Design review of the part built by this model. Coordinates are the model's own, in mm. A direction names the side the tool comes from. Give positions to 0.01 mm unless a question says otherwise; leave off trailing zeros. Write each loop counter-clockwise with the first axis right and the second up, starting at its lowest first coordinate (ties: lowest second). Pieces come first, ordered by that corner, then holes. Notation, with made-up numbers: M 3.5,89.25 L 42.5,89.25 A19 cw 42.5,117.25 Z; hole C 13,-12 d5. An arc over 180 degrees is marked long. Write each question's results on one line, items separated by ' | '. Start each with the question number.
from build123d import *

# Parameters (mm, degrees)
SKETCH2_W               = 900
SKETCH2_H               = 300
BOSS_EXTRUDE1_DEPTH     = 600
CUT_EXTRUDE1_DEPTH      = 1
CUT_EXTRUDE1_DEPTH_BACK = 900
CUT_EXTRUDE2_DEPTH      = 1
CUT_EXTRUDE2_DEPTH_BACK = 598.5
SKETCH6_W               = 897
SKETCH6_H               = 597
CUT_EXTRUDE4_DEPTH      = 48.5


with BuildPart() as part:
    # Sketch2 → Boss-Extrude1 (new body)
    with BuildSketch(Plane.XY):
        with Locations((75.531914894, 52.659574468)):
            Rectangle(SKETCH2_W, SKETCH2_H)
    extrude(amount=-BOSS_EXTRUDE1_DEPTH)

    # Sketch3 → Cut-Extrude1 (cut, two sides)
    with BuildSketch(Plane.ZY.offset(374.468085106)) as cut_extrude1_sk:
        Polygon((-1951.6407865, 202.659574468), (-600, 202.659574468), (-598.5, 202.659574468), (-598.5, 52.659574468), (0, 52.659574468), (1351.6407865, 52.659574468), (1474.268787585, 2753.15834993), (-1829.012785414, 2903.15834993), align=None)
    extrude(amount=CUT_EXTRUDE1_DEPTH, mode=Mode.SUBTRACT)
    extrude(cut_extrude1_sk.sketch, amount=-CUT_EXTRUDE1_DEPTH_BACK, mode=Mode.SUBTRACT)

    # Sketch4 → Cut-Extrude2 (cut, two sides)
    with BuildSketch(Plane.XY) as cut_extrude2_sk:
        Polygon((-2209.296844196, 52.659574468), (-374.468085106, 52.659574468), (-372.968085106, 52.659574468), (-372.968085106, -47.340425532), (524.031914894, -47.340425532), (524.031914894, 52.659574468), (525.531914894, 52.659574468), (2360.360673983, 52.659574468), (2360.360673983, 3722.317092647), (-2209.296844196, 3722.317092647), align=None)
    extrude(amount=CUT_EXTRUDE2_DEPTH, mode=Mode.SUBTRACT)
    extrude(cut_extrude2_sk.sketch, amount=-CUT_EXTRUDE2_DEPTH_BACK, mode=Mode.SUBTRACT)

    # Sketch6 → Cut-Extrude4 (cut)
    with BuildSketch(Plane(origin=(0, -47.340425532, 0), x_dir=(1, 0, 0), z_dir=(0, 1, 0))):
        with Locations((75.531914894, 300)):
            Rectangle(SKETCH6_W, SKETCH6_H)
    extrude(amount=-CUT_EXTRUDE4_DEPTH, mode=Mode.SUBTRACT)


solid = part.part
Q1. For pin 1 Ø1.2 at (x, z) = (-374, -239) entering from +Y; pin 2 Ø0.8 at (x, z) = (-17.5, -0.5) entering from +Y; pin 3 Ø1 at (x, z) = (256.5, -401.5) entering from +Y, all flat-tipped, find the tip position at first contact; note any pin that passes through.
Q2. We need section D-D on y = 139. Write out the cut boundary in (x, z).
Q3. The part is to be moulded in two halves that separate along X. For faces 1 (the flat face through (69, -95.84, -304)), 2 (the flat face through (525.532, -16, -296)), 3 (the flat face through (69, -97.34, -296)), say which applies: pulls with the +X half, pulls with the -X half, needs draft (parallel to the pull), parting line crosses it, or undercut.
Q4. Wall thickness on line 1 along X through (y, z) = (11, -353); line 2 along Z through (x, y) = (-227.5, -83); line 3 along Y through (x, z) = (48, -434.5): over which ranges is each line inside the solid? List them lowest first. Write a range as from..to.
Q5. We need section A-A on z = -544. Write out the cut boundary in (x, y), and give its area (3 significant figures).
Q6. We need section C-C on y = -73.5. Write out the cut boundary in (x, z).
Q7. We need section B-B on x = 383.5. Write out the cut boundary in (y, z).
Q8. For faces 4 (the flat face through (-372.968, -21, -295)), 5 (the flat face through (73, -66, 0)), list the 3-axis set-ups (+Z, -Z, +X, -X, +Y, -Y) from which the entire face can be reached by the end or side of a thin tool; tool diameter is ignored.
Answer sheet:
1) pin 1: y = 52.66 | pin 2: y = -47.34 | pin 3: y = -95.84
2) outline: M -374.47,-600 L 525.53,-600 L 525.53,-598.5 L -374.47,-598.5 Z
3) face 1: undercut | face 2: pulls with the +X half | face 3: needs draft
4) line 1: -374.47..-372.97, 524.03..525.53 | line 2: -600..-598.5, -1.5..0 | line 3: -97.34..-95.84
5) outline: M -374.47,-97.34 L 525.53,-97.34 L 525.53,52.66 L 524.03,52.66 L 524.03,-95.84 L -372.97,-95.84 L -372.97,52.66 L -374.47,52.66 Z | area: 1,800 mm^2
6) outline: M -374.47,-600 L 525.53,-600 L 525.53,0 L -374.47,0 Z; hole M -372.97,-598.5 L 524.03,-598.5 L 524.03,-1.5 L -372.97,-1.5 Z
7) outline: M -97.34,-600 L 202.66,-600 L 202.66,-598.5 L -95.84,-598.5 L -95.84,-1.5 L -47.34,-1.5 L -47.34,0 L -97.34,0 Z
8) face 4: +Y | face 5: +Z, +X, -X, +Y, -Y
